The listing builds one solid part. Answer for the finished solid, in the listing's coordinates (mm). Face numbers are marked on the shaded views. A direction names the side the tool comes from. Coordinates: 2 decimals unless noted, no trailing zeros. Write each loop counter-clockwise with the first axis right and the second up, starting at its lowest first coordinate (ties: lowest second). Pieces come first, ordered by that corner, then holes.
from build123d import *

# Parameters (mm, degrees)
F0_W     = 20
F0_H     = 55
F0_R     = 2
F0_R_2   = 2.5
F1_DEPTH = 10
F2_R     = 3.75
F3_DEPTH = 5
F4_W     = 20
F4_H     = 20
F4_R     = 2.5
F5_DEPTH = 3
F6_R     = 5
F7_R     = 4.75
F7_R_2   = 2.5
F8_DEPTH = 3


with BuildPart() as f1:
    # F0 (on Top) → F1 (new body)
    with BuildSketch(Plane.XY):
        with Locations((10, 27.5)):
            Rectangle(F0_W, F0_H)
        with Locations((10, 5)):
            Circle(F0_R, mode=Mode.SUBTRACT)
        with Locations((10, 30)):
            Circle(F0_R, mode=Mode.SUBTRACT)
        with Locations((10, 45)):
            Circle(F0_R_2, mode=Mode.SUBTRACT)
    extrude(amount=F1_DEPTH)

    # F2 (on face) → F3 (cut)
    with BuildSketch(Plane.XY.offset(10)):
        with Locations((10, 5)):
            Circle(F2_R)
        with Locations((10, 30)):
            Circle(F2_R)
    extrude(amount=-F3_DEPTH, mode=Mode.SUBTRACT)

    # F4 (on face) → F5 (cut)
    with BuildSketch(Plane.XY.offset(10)):
        with Locations((10, 45)):
            Rectangle(F4_W, F4_H)
        with Locations((10, 45)):
            Circle(F4_R, mode=Mode.SUBTRACT)
    extrude(amount=-F5_DEPTH, mode=Mode.SUBTRACT)

    # F6
    f6_edges = [f1.edges().sort_by_distance(p)[0] for p in [
        (20, 0, 5),
        (20, 55, 3.5),
        (0, 55, 3.5),
        (0, 0, 5),
        (20, 35, 8.5),
        (0, 35, 8.5),
    ]]
    fillet(f6_edges, radius=F6_R)

    # F7 (on face) → F8 (cut)
    with BuildSketch(Plane.XY):
        with Locations((10, 45)):
            Circle(F7_R)
        with Locations((10, 45)):
            Circle(F7_R_2, mode=Mode.SUBTRACT)
    extrude(amount=F8_DEPTH, mode=Mode.SUBTRACT)


solid = f1.part
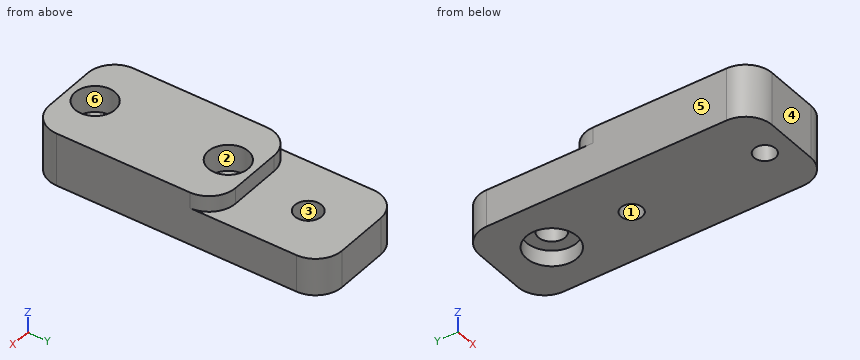
1. A tool of negligible diameter and unlimited length cuts with its end or side. For the marked faces 1 and 2, from which of +Z, -Z, +X, -X, +Y, -Y can it reach the whole face along a straight path? Write none if from no direction.
Results found:
face 1: +Z, -Z
face 2: +Z
2. Section D-D on y = 27 is taken. Give the vertices of the cut face in (x, z).
Results found:
outline: (0, 0) - (20, 0) - (20, 10) - (12.25, 10) - (12.25, 5) - (7.75, 5) - (7.75, 10) - (0, 10) - close
3. Find the intervals of material crossed by L1, parallel to Y at x = 10, z = 1.5; L2, parallel to Y at x = 10, z = 3.9; L3, parallel to X at y = 30, z = 2.3, in increasing order.
Results found:
L1: y = 0 to 3, 7 to 28, 32 to 40.25, 49.75 to 55
L2: y = 0 to 3, 7 to 28, 32 to 42.5, 47.5 to 55
L3: x = 0 to 8, 12 to 20
4. For a pull along X with two mould halves and no side action, classify the marked faces 3, 4, 5 and 6 as pulls with the +X half, pulls with the -X half, needs draft (parallel to the pull), parting line crosses it, or undercut.
Results found:
face 3: undercut
face 4: needs draft
face 5: pulls with the -X half
face 6: undercut
5. Section A-A on x = 10 is taken. State how many separate pieces and enclosed holes the cut face has, then the cut area to 4 significant figures.
Results found:
separate pieces: 4
enclosed holes: 0
area: 326.5 mm2
6. Flat-ended cylindrical pins translate along their axes: P1, Ø1.5, axis at y = 46.5, z = 9, coming from the +X side; P2, Ø5, axis at x = 10, y = 30, coming from the +Z side; P3, Ø7, axis at x = 10, y = 5, coming from the -Z side; P4, Ø3.5, axis at x = 11, z = 9, coming from the +Y side. Find the tip coordinate at first contact, or state that the pin passes through.
Results found:
P1: passes through
P2: stops at z = 5
P3: stops at z = 0
P4: stops at y = 35
7. Section B-B on z = 6 is taken. Give the vertices of the cut face in (x, y), then the cut area to 3 significant figures.
Results found:
outline: (0, 5) arc R5 ccw to (5, 0) - (15, 0) arc R5 ccw to (20, 5) - (20, 50) arc R5 ccw to (15, 55) - (5, 55) arc R5 ccw to (0, 50) - close; hole circle Ø7.5 at (10, 5); hole circle Ø7.5 at (10, 30); hole circle Ø5 at (10, 45)
area: 971 mm2
8. Section C-C on y = 45 is taken. Give the vertices of the cut face in (x, z), then the cut area to 3 significant figures.
Results found:
outline: (0, 0) - (5.25, 0) - (5.25, 3) - (7.5, 3) - (7.5, 7) - (0, 7) - close; (12.5, 3) - (14.75, 3) - (14.75, 0) - (20, 0) - (20, 7) - (12.5, 7) - close
area: 91.5 mm2
